Autodesk Inventor part; units mm, degrees
ref_plane "YZ Plane" through (0, 0, 0) normal (1, 0, 0) x (0, 1, 0)
ref_plane "XZ Plane" through (0, 0, 0) normal (0, 1, 0) x (-1, 0, 0)
ref_plane "XY Plane" through (0, 0, 0) normal (0, 0, 1) x (1, 0, 0)
sketch "Sketch1" plane through (0, 0, 0) normal (0, 0, 1) x (1, 0, 0)
  line L0 (-15.7, 12.7) -> (-12.7, 12.7)
  line L1 (-12.7, 12.7) -> (-12.7, -9.7)
  line L2 (-12.7, -9.7) -> (12.7, -9.7)
  line L3 (12.7, -9.7) -> (12.7, 12.7)
  line L4 (12.7, 12.7) -> (15.7, 12.7)
  line L5 (15.7, 12.7) -> (15.7, -12.7)
  line L6 (15.7, -12.7) -> (-15.7, -12.7)
  line L7 (-15.7, -12.7) -> (-15.7, 12.7)
  point P0 (0, 0)
  dimension "d0" = 3
  dimension "d2" = 3
  dimension "d3" = 25.4
  dimension "d4" = 31.4
  dimension "d5" = 15.7
  dimension "d7" = 12.7
  dimension "d8" = 3
extrude "Extrusion1" add sketch "Sketch1" against normal blind 660.4
sketch "Sketch5" plane through (15.7, -12.7, 0) normal (1, 0, 0) x (0, 0, -1)
  circle A0 centre (13.8784, 12.3) radius 3.175
  circle A1 centre (91.9, 12.3) radius 3.175
  circle A2 centre (168.1, 12.3) radius 3.175
  circle A3 centre (244.3, 12.3) radius 3.175
  circle A4 centre (320.5, 12.3) radius 3.175
  circle A5 centre (396.7, 12.3) radius 3.175
  circle A6 centre (472.9, 12.3) radius 3.175
  circle A7 centre (549.1, 12.3) radius 3.175
  circle A8 centre (645.6513, 12.3) radius 3.175
  point P0 (0, 12.7)
  dimension "d56" = 6.35
  dimension "d58" = 6.35
  dimension "d59" = 6.35
  dimension "d60" = 6.35
  dimension "d61" = 6.35
  dimension "d62" = 6.35
  dimension "d63" = 6.35
  dimension "d64" = 6.35
  dimension "d65" = 6.35
extrude "Extrusion5" cut sketch "Sketch5" against normal blind 76.2
equation "\"d2\" = d0"
equation "\"d8\" = d0"
equation "\"d58\" = d56"
equation "\"d59\" = d58"
equation "\"d60\" = d59"
equation "\"d61\" = d60"
equation "\"d62\" = d61"
equation "\"d63\" = d62"
equation "\"d64\" = d63"
equation "\"d65\" = d64"
properties part number "26in C-Channel Left" material "Aluminum 6061"
The listing builds one solid part. Answer for the finished solid, in the listing's coordinates (mm). A direction names the side the tool comes from. Coordinates: 2 decimals unless noted, no trailing zeros. Write each loop counter-clockwise with the first axis right and the second up, starting at its lowest first coordinate (ties: lowest second). Pieces come first, ordered by that corner, then holes. Notation, with made-up numbers: (44.25, 52) - (82.25, 52) arc R32 cw to (82.25, 87) - close; hole circle Ø7 at (19, -33.5). An arc over 180 degrees is marked (long way). Put each result on its own line as item: value.
1. Flat-ended cylindrical pins translate along their axes: pin 1 Ø6 at (x, z) = (2.5, -497) entering from +Y; pin 2 Ø6 at (x, y) = (7, -2.5) entering from +Z. Find the tip coordinate at first contact, or state that the pin passes through.
Answer sheet:
pin 1: stops at y = -9.7
pin 2: passes through
2. The part is cut by section A-A on z = -531.5. Give the vertices of the cut face in (x, y).
Answer sheet:
outline: (-15.7, -12.7) - (15.7, -12.7) - (15.7, 12.7) - (12.7, 12.7) - (12.7, -9.7) - (-12.7, -9.7) - (-12.7, 12.7) - (-15.7, 12.7) - close
3. Find the intervals of material crossed by line 1 along X through (y, z) = (0.75, -479); line 2 along Y through (x, z) = (-13.4, -168.1) (3 decimals); line 3 along Y through (x, z) = (-8.5, -169.5), in increasing order. Write a range as from..to.
Answer sheet:
line 1: x = -15.7..-12.7, 12.7..15.7
line 2: y = -12.7..-3.575, 2.775..12.7
line 3: y = -12.7..-9.7
4. A tool of negligible diameter and unlimited length cuts with its end or side. For faces 1 (the face through (0, -10, 0)), 2 (the face through (0, -9.7, -326)), from which of +Z, -Z, +X, -X, +Y, -Y can it reach the whole face along a straight path? Write none if from no direction.
Answer sheet:
face 1: +Z, +X, -X, +Y, -Y
face 2: +Z, -Z, +Y
5. Determine the mould class of faces 3 (the face through (12.7, 1, -326)), 4 (the face through (15.7, 0, -326)), 5 (the face through (0, -10, -660.4)) for opening direction X: pulls with the +X half, pulls with the -X half, needs draft (parallel to the pull), parting line crosses it, or undercut.
Answer sheet:
face 3: undercut
face 4: pulls with the +X half
face 5: needs draft
6. The part is cut by section B-B on x = -1. Give the vertices of the cut face in (y, z).
Answer sheet:
outline: (-12.7, -660.4) - (-9.7, -660.4) - (-9.7, 0) - (-12.7, 0) - close
